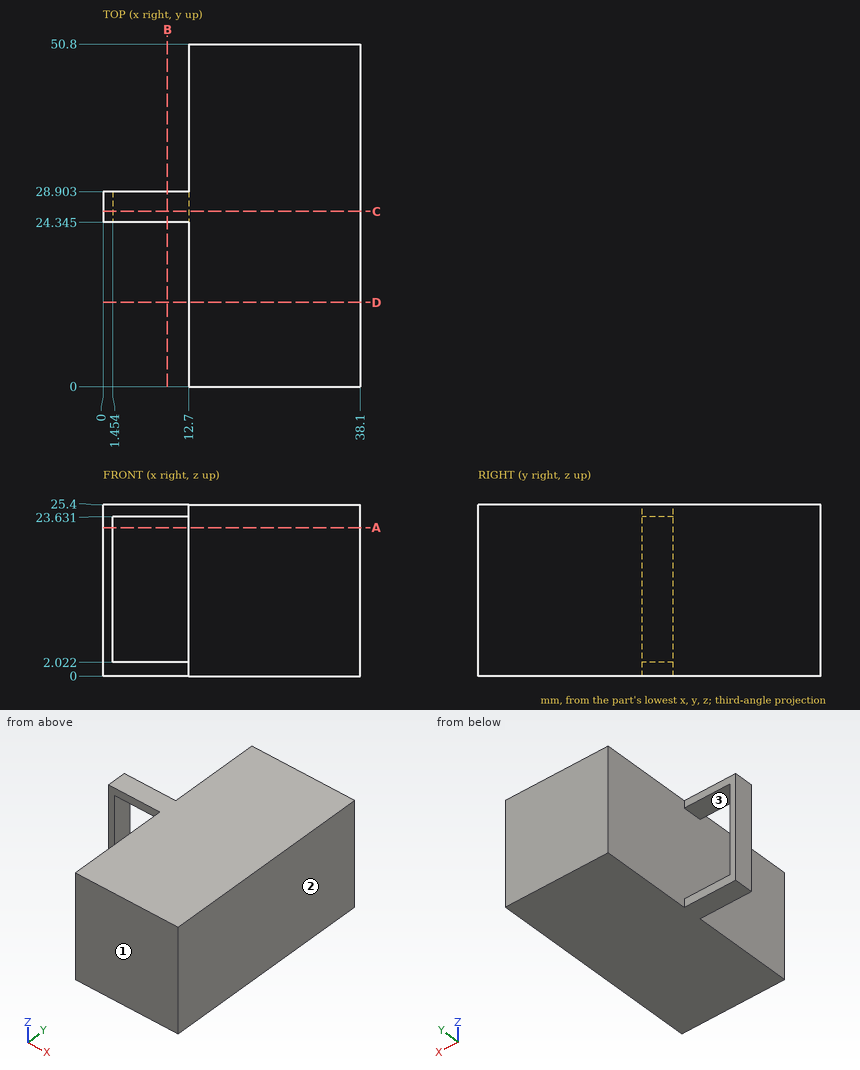
Can you work these out from the drawing? Everything is in mm from the part's minimum corner. Coordinates: 2 decimals unless noted, no trailing zeros. Order: outer loops, then holes, each group sorted by start corner. A loop starts at its lowest first (then second) coordinate and runs counter-clockwise, first axis right, second up. Notation, with made-up numbers: M -37.75,63.25 L 18.25,63.25 A25 cw 18.25,96.25 Z; hole C 76.5,44.5 d8. An arc over 180 degrees is marked long. Answer as CSV lines item,"result". Start each with the question number.
1. I want a section at A-A, the plane z = 22. Write out the boundary of the cut face in (x, y) (1 decimal).
2. For pin 1 (1.5 mm diameter, centred on x = 25.5, z = 11.5, fed in from -Y); pin 2 (2 mm diameter, centred on y = 40.5, z = 20.5, fed in from -X), each with a flat end and sliding along its axis, tell me the tip position at first contact or that it passes through.
3. We'd pull the mould along X, two halves only. Please class the marked faces 1, 2 and 3: released by +X, released by -X, zero draft, split by the parting line, or undercut.
4. I need wall thicknesses on line 1 (Z direction, x = 6.5, y = 27.5); line 2 (X direction, y = 12, z = 6.25). Which ranges of each line are inside material? Lowest first, please. Write a range as [from, to].
5. I want a section at B-B, the plane x = 9.5. Write out the boundary of the cut face in (y, z) (1 decimal), and give its area (3 significant figures).
6. I want a section at D-D, the plane y = 12.5. Write out the boundary of the cut face in (x, z).
7. I want a section at C-C, the plane y = 26. Write out the boundary of the cut face in (x, z) (1 decimal), and give its area (3 significant figures).
Recorded:
1,outline,"M 0,24.3 L 1.5,24.3 L 1.5,28.9 L 0,28.9 Z; M 12.7,0 L 38.1,0 L 38.1,50.8 L 12.7,50.8 Z"
2,pin 1,"stops at y = 0"
2,pin 2,"stops at x = 12.7"
3,face 1,"zero draft"
3,face 2,"released by +X"
3,face 3,"undercut"
4,line 1,"z = [0, 2.02], [23.63, 25.4]"
4,line 2,"x = [12.7, 38.1]"
5,outline,"M 24.3,0 L 28.9,0 L 28.9,2 L 24.3,2 Z; M 24.3,23.6 L 28.9,23.6 L 28.9,25.4 L 24.3,25.4 Z"
5,area,"17.3 mm2"
6,outline,"M 12.7,0 L 38.1,0 L 38.1,25.4 L 12.7,25.4 Z"
7,outline,"M 0,0 L 38.1,0 L 38.1,25.4 L 0,25.4 Z; hole M 1.5,2 L 12.7,2 L 12.7,23.6 L 1.5,23.6 Z"
7,area,"725 mm2"
